Verification items for this drawing (mm, ordinates from the low corner). A direction names the side the tool comes from. Round coordinates to 2 decimals unless told otherwise and drop trailing zeros. Loops run counter-clockwise (first coordinate to the right, second up) from the corner with the lowest first, then second, coordinate; pieces in that order, holes last. Notation, with made-up numbers: (59.25, 15.25) - (83.25, 15.25) arc R26 cw to (83.25, 50.25) - close; hole circle Ø3 at (-33, -10). An arc over 180 degrees is marked (long way). Answer in a Markdown table with one row per item. Add a question column.
(1) Thickness scan on line 1 along Z through (x, y) = (249, 32); line 2 along X through (y, z) = (14.5, 97.5). Record the ranges inside material, lowest first.
(2) Cross-section at B-B on y = 23.5. Enter the section's corners in (x, z), then the cut area to 3 significant figures.
(3) Access from +Z, -Z, +X, -X, +Y, -Y to the whole of each face (thin tool, end or side, straight path). Record for the marked faces 1 and 2.
(4) Cross-section at A-A on x = 56. Enter the section's corners in (y, z), then the cut area to 3 significant figures.
(5) Cross-section at C-C on z = 149. Enter the section's corners in (x, y), then the cut area to 3 significant figures.
(6) Gauge pin test, flat end, axial feed: pin 1 (19 mm diameter, centred on y = 24.5, z = 115, fed in from -X). Record the tip position at first contact, or that the pin passes through.
(7) Mould release check, pull along Z, two halves, no side actions. Record for the marked faces 3, 4 and 5: +Z half, -Z half, draft (parallel to the pull), parting line (faces both ways), or undercut.
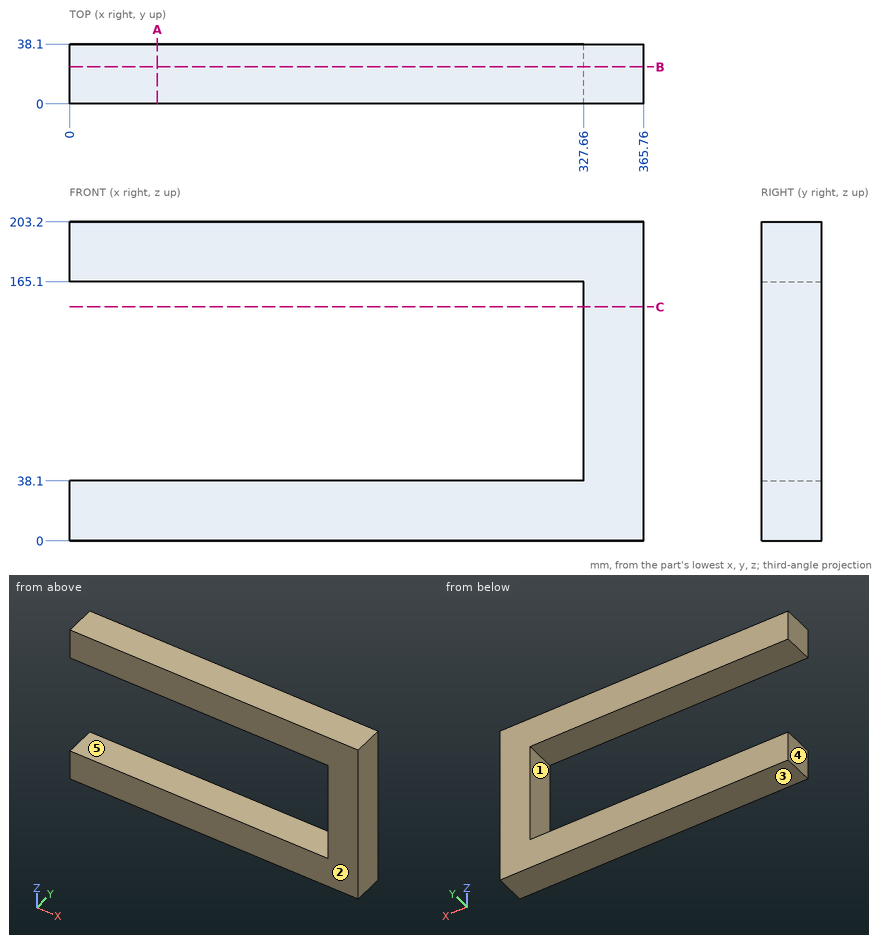
Answers:
| question | item | result |
|---|---|---|
| 1 | line 1 | z = 0 to 38.1, 165.1 to 203.2 |
| 1 | line 2 | x = 327.66 to 365.76 |
| 2 | outline | (0, 0) - (365.76, 0) - (365.76, 203.2) - (0, 203.2) - (0, 165.1) - (327.66, 165.1) - (327.66, 38.1) - (0, 38.1) - close |
| 2 | area | 32,700 mm^2 |
| 3 | face 1 | -X, +Y, -Y |
| 3 | face 2 | +Z, -Z, +X, -X, -Y |
| 4 | outline | (0, 0) - (38.1, 0) - (38.1, 38.1) - (0, 38.1) - close; (0, 165.1) - (38.1, 165.1) - (38.1, 203.2) - (0, 203.2) - close |
| 4 | area | 2,900 mm^2 |
| 5 | outline | (327.66, 0) - (365.76, 0) - (365.76, 38.1) - (327.66, 38.1) - close |
| 5 | area | 1,450 mm^2 |
| 6 | pin 1 | stops at x = 327.66 |
| 7 | face 3 | -Z half |
| 7 | face 4 | draft |
| 7 | face 5 | undercut |
